```python
from build123d import *

# Parameters (mm, degrees)
SKETCH_1_R          = 6.9
EXTRUDE_1_DEPTH     = 4
SKETCH_2_R          = 5.817135152
SKETCH_2_R_2        = 2.2
CUT_EXTRUDE_2_DEPTH = 3.2
SKETCH_3_R          = 1.5
CUT_EXTRUDE_3_DEPTH = 11.546089323


with BuildPart() as part:
    # Эскиз1 → Вытянуть1 (new body)
    with BuildSketch(Plane(origin=(0, 0, 0), x_dir=(1, 0, 0), z_dir=(0, 1, 0))):
        with Locations(Location((0, 0, 0), (0, 0, 270))):
            Circle(SKETCH_1_R)
    extrude(amount=EXTRUDE_1_DEPTH)

    # Эскиз2 → Вытянуть2 (cut)
    with BuildSketch(Plane(origin=(0, 4, 0), x_dir=(1, 0, 0), z_dir=(0, 1, 0))):
        with Locations(Location((0, 0, 0), (0, 0, 270))):
            Circle(SKETCH_2_R)
        with Locations(Location((0, 0, 0), (0, 0, 270))):
            Circle(SKETCH_2_R_2, mode=Mode.SUBTRACT)
    extrude(amount=-CUT_EXTRUDE_2_DEPTH, mode=Mode.SUBTRACT)

    # Эскиз3 → Вытянуть3 (cut, through all)
    with BuildSketch(Plane(origin=(0, 4, 0), x_dir=(1, 0, 0), z_dir=(0, 1, 0))):
        with Locations(Location((0, 0, 0), (0, 0, 270))):
            Circle(SKETCH_3_R)
    extrude(amount=-CUT_EXTRUDE_3_DEPTH, mode=Mode.SUBTRACT)


solid = part.part
```
Input: part model. Units: mm. Frame: model coordinates. A direction names the side the tool comes from. Give positions to 0.01 mm unless a question says otherwise; leave off trailing zeros. Order: outer loops, then holes, each group sorted by start corner. A loop starts at its lowest first (then second) coordinate and runs counter-clockwise, first axis right, second up. Notation, with made-up numbers: M 38.25,52.25 L 75.25,52.25 A30 cw 75.25,77.25 Z; hole C 65,31.5 d11. An arc over 180 degrees is marked long. One line per question, with ' | ' between items. Start each with the question number.
1. First-contact query: pin 1 Ø5 at (x, z) = (0.5, 5) entering from -Y; pin 2 Ø1.5 at (x, y) = (4.5, 0.5) entering from -Z. Flat tips, straight axial feed; report the tip coordinate or a pass-through.
2. Section query B-B (x = 0). Return the cut outline in (y, z), and give its area (3 significant figures).
3. Section query A-A (z = 0). Return the cut outline in (x, y).
4. Material intervals for probe 1 along X at (y, z) = (2.75, 0); probe 2 along X at (y, z) = (2.05, 1.25); probe 3 along Y at (x, z) = (5, -0.75), sorted ascending. Write a range as [from, to].
5. Section query D-D (x = -2.75). Return the cut outline in (y, z).
6. Access query for faces 4 (the face through (-5.68, 2.42, -1.26)), 5 (the face through (-5, 4, -4)). Directions: +Z, -Z, +X, -X, +Y, -Y. A direction counts if a zero-diameter tool reaches every point of the face in a straight line with its end or side. Return the directions, or none.
7. Section query C-C (y = 1.25). Return the cut outline in (x, z).
8. Pull-direction query (Z, two-part tool) for faces 1 (the face through (4.66, 1.97, -5.09)), 2 (the face through (0, 0.8, 3)), 3 (the face through (2, 0, 0)); classes: released by +Z, released by -Z, zero draft, split by the parting line, or undercut.
Here are the results:
1) pin 1: y = 0 | pin 2: z = -5.79
2) outline: M 0,-6.9 L 4,-6.9 L 4,-5.82 L 0.8,-5.82 L 0.8,-2.2 L 4,-2.2 L 4,-1.5 L 0,-1.5 Z; M 0,1.5 L 4,1.5 L 4,2.2 L 0.8,2.2 L 0.8,5.82 L 4,5.82 L 4,6.9 L 0,6.9 Z | area: 20.1 mm²
3) outline: M -6.9,0 L -1.5,0 L -1.5,4 L -2.2,4 L -2.2,0.8 L -5.82,0.8 L -5.82,4 L -6.9,4 Z; M 1.5,0 L 6.9,0 L 6.9,4 L 5.82,4 L 5.82,0.8 L 2.2,0.8 L 2.2,4 L 1.5,4 Z
4) probe 1: [-6.9, -5.82], [-2.2, -1.5], [1.5, 2.2], [5.82, 6.9] | probe 2: [-6.79, -5.68], [-1.81, -0.83], [0.83, 1.81], [5.68, 6.79] | probe 3: [0, 0.8]
5) outline: M 0,-6.33 L 4,-6.33 L 4,-5.13 L 0.8,-5.13 L 0.8,5.13 L 4,5.13 L 4,6.33 L 0,6.33 Z
6) face 4: +Y | face 5: +Z, -Z, +X, -X, +Y
7) outline: C 0,0 d13.8; C 0,0 d4.4; hole C 0,0 d11.63; hole C 0,0 d3
8) face 1: split by the parting line | face 2: undercut | face 3: zero draft
